from build123d import *
from OCP.BRepFilletAPI import BRepFilletAPI_MakeFillet

# Parameters (mm, degrees)
BOSS_EXTRUDE1_DEPTH = 37.5
SKETCH2_R           = 1.5
SKETCH2_R_2         = 1.85
CUT_EXTRUDE1_DEPTH  = 56.192843739
FILLET1_R1          = 4
FILLET1_R2          = 10


with BuildPart() as part:
    # Sketch1 → Boss-Extrude1 (new, symmetric)
    with BuildSketch(Plane.XY):
        Polygon((-34, 18), (-15, 18), (-15, 0), (15, 0), (15, 18), (34, 18), (34, 14), (19, 14), (19, -4), (-19, -4), (-19, 14), (-34, 14), align=None)
    extrude(amount=BOSS_EXTRUDE1_DEPTH, both=True)

    # Sketch2 → Cut-Extrude1 (cut, through all)
    with BuildSketch(Plane.XZ.offset(4)):
        with Locations((0, 22.5)):
            Circle(SKETCH2_R)
        with Locations((0, -22.5)):
            Circle(SKETCH2_R)
        with Locations((-26.5, 27.5)):
            Circle(SKETCH2_R_2)
        with Locations((-26.5, 0)):
            Circle(SKETCH2_R_2)
        with Locations((-26.5, -27.5)):
            Circle(SKETCH2_R_2)
        with Locations((26.5, 27.5)):
            Circle(SKETCH2_R_2)
        with Locations((26.5, -27.5)):
            Circle(SKETCH2_R_2)
        with Locations((26.5, 0)):
            Circle(SKETCH2_R_2)
    extrude(amount=-CUT_EXTRUDE1_DEPTH, mode=Mode.SUBTRACT)

    # Fillet1: one fillet with a radius per group of edges: ONE call of the kernel's fillet builder (fillet() takes one radius for all edges)
    fillet1_edges_1 = [part.edges().sort_by_distance(p)[0] for p in [
        (-15, 0, 0),
        (15, 0, 0),
        (-19, -4, 0),
        (19, -4, 0),
        (19, 14, 0),
        (-19, 14, 0),
    ]]
    fillet1_edges_2 = [part.edges().sort_by_distance(p)[0] for p in [
        (-34, 16, 37.5),
        (-34, 16, -37.5),
        (34, 16, -37.5),
        (34, 16, 37.5),
    ]]
    fillet1 = BRepFilletAPI_MakeFillet(part.part.solid().wrapped)
    for e in fillet1_edges_1:
        fillet1.Add(FILLET1_R1, e.wrapped)
    for e in fillet1_edges_2:
        fillet1.Add(FILLET1_R2, e.wrapped)
    add(Compound.cast(fillet1.Shape()), mode=Mode.REPLACE)


solid = part.part
Model file for the job. Use its own axes, mm. A direction names the side the tool comes from. Coordinates: 2 decimals unless noted, no trailing zeros. Write each loop counter-clockwise with the first axis right and the second up, starting at its lowest first coordinate (ties: lowest second). Pieces come first, ordered by that corner, then holes. Notation, with made-up numbers: (20.25, 24.5) -> (43.25, 24.5) arc R13 cw to (43.25, 33.5) -> close; hole circle Ø5 at (-5, -17.75). An arc over 180 degrees is marked (long way). One line per item, written item: value. Start each with the question number.
1) Probe probe 1 along Z at (x, y) = (0, -1.5); probe 2 along X at (y, z) = (6, -4); probe 3 along Z at (x, y) = (-26.5, 15.25). List the from-to ranges inside material, lowest first.
2) Pull direction X, two halves, no side cores. Call faces 3 (the face through (0, -2, 24)), 4 (the face through (-30, 14, 1)), 5 (the face through (-17.797, -2.859, -0.525)): +X half, -X half, draft (parallel to the pull), parting line (faces both ways), or undercut.
3) Slice it at B-B on y = 9. Write the cut outline in (x, z).
4) Slice it at C-C on x = 0. Write the cut outline in (y, z), then the cut area to 3 significant figures.
5) Slice it at D-D on x = -26. Write the cut outline in (y, z).
6) Flat gauge pins, fed straight in: pin 1 Ø6 at (y, z) = (2, -2.5) entering from -X; pin 2 Ø4 at (x, z) = (0, 22.5) entering from -Y; pin 3 Ø4 at (x, z) = (0, -22.5) entering from +Y; pin 4 Ø5 at (x, z) = (26.5, 0) entering from -Y. Where does each tip first touch, or does it go through?
7) Slice it at A-A on z = 22.5. Write the cut outline in (x, y).
8) Which spindle directions (+Z, -Z, +X, -X, +Y, -Y) get a long thin tool onto all of the face, cutting with end or side? Do faces 1 (the face through (15, 11, 1)), 2 (the face through (25.136, 15.972, 28.75)). Say none if no direction does.
Answers follow:
1. probe 1: -37.5 to -24, -21 to 21, 24 to 37.5
1. probe 2: -19 to -15, 15 to 19
1. probe 3: -37.18 to -29.35, -25.65 to -1.85, 1.85 to 25.65, 29.35 to 37.18
2. face 3: undercut
2. face 4: draft
2. face 5: -X half
3. outline: (-19, -37.5) -> (-15, -37.5) -> (-15, 37.5) -> (-19, 37.5) -> close; (15, -37.5) -> (19, -37.5) -> (19, 37.5) -> (15, 37.5) -> close
4. outline: (-4, -37.5) -> (0, -37.5) -> (0, -24) -> (-4, -24) -> close; (-4, -21) -> (0, -21) -> (0, 21) -> (-4, 21) -> close; (-4, 24) -> (0, 24) -> (0, 37.5) -> (-4, 37.5) -> close
4. area: 276 mm2
5. outline: (14, -37.3) -> (18, -37.3) -> (18, -29.28) -> (14, -29.28) -> close; (14, -25.72) -> (18, -25.72) -> (18, -1.78) -> (14, -1.78) -> close; (14, 1.78) -> (18, 1.78) -> (18, 25.72) -> (14, 25.72) -> close; (14, 29.28) -> (18, 29.28) -> (18, 37.3) -> (14, 37.3) -> close
6. pin 1: x = -19
6. pin 2: y = -4
6. pin 3: y = 0
6. pin 4: y = 14
7. outline: (-34, 14) -> (-23, 14) arc R4 cw to (-19, 10) -> (-19, 0) arc R4 ccw to (-15, -4) -> (-1.5, -4) -> (-1.5, 0) -> (-11, 0) arc R4 cw to (-15, 4) -> (-15, 18) -> (-34, 18) -> close; (1.5, -4) -> (15, -4) arc R4 ccw to (19, 0) -> (19, 10) arc R4 cw to (23, 14) -> (34, 14) -> (34, 18) -> (15, 18) -> (15, 4) arc R4 cw to (11, 0) -> (1.5, 0) -> close
8. face 1: +Z, -Z, +Y
8. face 2: +Y, -Y
